Autodesk Fusion 360 part; units mm, degrees
sketch "Esquisse1" plane through (0, 0, 0) normal (0, 1, 0) x (1, 0, 0)
  circle A0 centre (0, 0) radius 42.5
  dimension "d1" = 85
extrude "Extrusion1" add sketch "Esquisse1" along normal blind 12
sketch "Esquisse2" plane through (0, 0, 0) normal (0, -1, 0) x (1, 0, 0)
  circle A0 centre (0, 0) radius 42.5
  circle A1 centre (0, 0) radius 21.5
  dimension "d4" = 43
extrude "Extrusion2" add sketch "Esquisse2" along normal blind 14.5 contours A1
sketch "Esquisse3" plane through (0, -14.5, 0) normal (0, -1, 0) x (1, 0, 0)
  circle A0 centre (0, 0) radius 21.5
  circle A1 centre (0, 0) radius 3.1
  dimension "d7" = 6.2
extrude "Extrusion3" cut sketch "Esquisse3" against normal blind 30 contours A1
chamfer "Chanfrein1" distance 1.5 distance2 21 1 edges at (-39.6239, 0, 15.3687) measured on face at (42.4472, 8, 2.1185)
sketch "Esquisse4" plane through (0, 0, 0) normal (0, -1, 0) x (1, 0, 0)
  circle A0 centre (0, 0) radius 42.5
  circle A1 centre (0, 0) radius 42.5
  line L0 (-21.5, 0) -> (-21.4682, 36.6792)
  line L1 (-21.5, 0) -> (-21.472, -36.677)
  line L2 (21.5, 36.6606) -> (21.5, 0)
  line L3 (21.5, 0) -> (21.5109, -36.6542)
extrude "Extrusion4" cut sketch "Esquisse4" against normal blind 30 contours A0 A1 L2 L3 | A0 A1 L0 L1
sketch "Esquisse5" plane through (0, 12, 0) normal (0, 1, 0) x (-1, 0, 0)
  circle A0 centre (0, 0) radius 3.1
  line L0 (-21.5, 36.6606) -> (-21.5, 0)
  line L1 (-21.5, 0) -> (-21.5109, -36.6542)
  arc A1 (-21.5109, -36.6542) -> (21.472, -36.677) centre (0, 0) ccw
  line L2 (21.472, -36.677) -> (21.5, 0)
  line L3 (21.5, 0) -> (21.4682, 36.6792)
  arc A2 (21.4682, 36.6792) -> (-21.5, 36.6606) centre (0, 0) ccw
  circle A3 centre (0, 0) radius 9.1
  dimension "d18" = 18.2
extrude "Extrusion5" cut sketch "Esquisse5" against normal blind 7 contours A3
fillet "Congé1" radius 2 6 edges at (21.5, 12, 18.3303) (21.5055, 12, -18.3271) (0.0226, 12, -42.5) (-21.486, 12, -18.3385) (-21.4841, 12, 18.3396) (0.0184, 12, 42.5)
Input: part model. Units: mm. Frame: model coordinates. A direction names the side the tool comes from. Give positions to 0.01 mm unless a question says otherwise; leave off trailing zeros. Write each loop counter-clockwise with the first axis right and the second up, starting at its lowest first coordinate (ties: lowest second). Pieces come first, ordered by that corner, then holes. Notation, with made-up numbers: M 14,9 L 56,9 A24 ccw 56,41 Z; hole C 73.25,78.25 d11. An arc over 180 degrees is marked long. Write item = value, one per line. Start each with the question number.
1) First-contact query: pin 1 Ø5 at (y, z) = (2, -10) entering from +X; pin 2 Ø3 at (x, y) = (15.5, -5) entering from +Z; pin 3 Ø8 at (x, z) = (0, 0) entering from +Y. Flat tips, straight axial feed; report the tip coordinate or a pass-through.
2) Draft query along Z for faces 3 (the cylindrical face through (-2.799, -7.148, -21.317)), 4 (the flat face through (0, 5, -4)), 5 (the cylindrical face through (-21.19, 5.77, -36.54)). Return one class per face: +Z half, -Z half, draft (parallel to the pull), parting line (faces both ways), or undercut.
3) Cut plane A-A on y = -1. Return the cut outline in (x, z).
4) Material intervals for line 1 along Z through (x, y) = (0, -1.5); line 2 along Z through (x, y) = (0, 7); line 3 along X through (y, z) = (8.5, -18.5), sorted ascending. Write a range as [from, to].
5) Reachability of faces 1 (the conical face through (-0.584, 0.427, 27.477)), 2 (the cylindrical face through (1.973, 8.549, -8.884)) from +Z, -Z, +X, -X, +Y, -Y: full face, straight path, thin tool, end or side. Return the list, or none.
Solved:
q1.pin_1 = 21.5
q1.pin_2 = 16.32
q1.pin_3 = 5
q2.face_3 = parting line
q2.face_4 = undercut
q2.face_5 = -Z half
q3.outline = C 0,0 d43; hole C 0,0 d6.2
q4.line_1 = [-21.5, -3.1], [3.1, 21.5]
q4.line_2 = [-42.5, -9.1], [9.1, 42.5]
q4.line_3 = [-21.49, 21.51]
q5.face_1 = +Z, -Y
q5.face_2 = +Y
